from build123d import *

# Parameters (mm, degrees)
F0_R      = 57.15
F0_R_2    = 54.61
F1_DEPTH  = 12.7
F2_R      = 57.15
F2_R_2    = 55.88
F3_DEPTH  = 6.35
F5_DEPTH  = 25.4
F6_R      = 10.16
F8_R      = 57.3643246116
F8_R_2    = 56.3769302999
F9_DEPTH  = 5.08
F11_SIZE  = 3.81
F12_R     = 30.0710840357
F13_DEPTH = 5.08


# Not quite as in the source:
# - a fillet or chamfer that OpenCascade refuses, or shapes differently, is made with other operations: its cross-section is extruded or revolved along the edge and cut away or added
# - a feature names something its author has since deleted; it is built from what else it names


with BuildPart() as f1:
    # F0 (on Front) → F1 (new body)
    with BuildSketch(Plane.XZ):
        Circle(F0_R)
        Circle(F0_R_2, mode=Mode.SUBTRACT)
        Circle(F0_R_2)
    extrude(amount=F1_DEPTH)

    # F2 (on face) → F3 (join)
    with BuildSketch(Plane.XZ.offset(12.7)):
        Circle(F2_R)
        Circle(F2_R_2, mode=Mode.SUBTRACT)
    extrude(amount=F3_DEPTH)

    # F4 (on face) → F5 (join)
    with BuildSketch(Plane.XZ.offset(12.7)):
        with BuildLine():
            Line((9.1685925479, 8.7878843126), (12.836029567, 12.3030380376))
            ThreePointArc((12.836029567, 12.3030380376), (6.9778357566, 16.3535380928), (0, 17.78))
            Line((0, 17.78), (0, 12.7))
            ThreePointArc((0, 12.7), (4.9841683976, 11.6810986377), (9.1685925479, 8.7878843126))
        make_face()
        with BuildLine():
            ThreePointArc((12.3030380376, -12.836029567), (16.3535380928, -6.9778357566), (17.78, 0))
            Line((17.78, 0), (12.7, 0))
            ThreePointArc((12.7, 0), (11.6810986377, -4.9841683976), (8.7878843126, -9.1685925479))
            Line((8.7878843126, -9.1685925479), (12.3030380376, -12.836029567))
        make_face()
        with BuildLine():
            ThreePointArc((-12.836029567, -12.3030380376), (-6.9778357566, -16.3535380928), (0, -17.78))
            Line((0, -17.78), (0, -12.7))
            ThreePointArc((0, -12.7), (-4.9841683976, -11.6810986377), (-9.1685925479, -8.7878843126))
            Line((-9.1685925479, -8.7878843126), (-12.836029567, -12.3030380376))
        make_face()
        with BuildLine():
            Line((-8.7878843126, 9.1685925479), (-12.3030380376, 12.836029567))
            ThreePointArc((-12.3030380376, 12.836029567), (-16.3535380928, 6.9778357566), (-17.78, 0))
            Line((-17.78, 0), (-12.7, 0))
            ThreePointArc((-12.7, 0), (-11.6810986377, 4.9841683976), (-8.7878843126, 9.1685925479))
        make_face()
    extrude(amount=F5_DEPTH)

    # F6
    f6_edges = [f1.edges().sort_by_distance(p)[0] for p in [
        (-57.15, 0, 0),
    ]]
    fillet(f6_edges, radius=F6_R)

    # F8 (on offset) → F9 (cut)
    with BuildSketch(Plane.XZ.offset(12.7)):
        Circle(F8_R)
        Circle(F8_R_2, mode=Mode.SUBTRACT)
    extrude(amount=F9_DEPTH, mode=Mode.SUBTRACT)

    # F10: fillet of radius 3.81 on 3 edges, made by hand

    # F10_s1 → F10_t2 (revolve)
    with BuildSketch(Plane.XY):
        with BuildLine():
            ThreePointArc((56.3769302999, -15.0006856268), (56.5753652345, -13.7871380263), (57.15, -12.7))
            Line((57.15, -12.7), (57.089261394, -12.6539862875))
            ThreePointArc((57.089261394, -12.6539862875), (56.7634651499, -12.6238), (56.3769302999, -12.6238))
            Line((56.3769302999, -12.6238), (56.3007302999, -12.7))
            Line((56.3007302999, -12.7), (56.3007302999, -15.0006856268))
            Line((56.3007302999, -15.0006856268), (56.3769302999, -15.0006856268))
        make_face()
    revolve(axis=Axis((0, -12.7, 0), (0, -1, 0)))

    # F10_s3 → F10_t4 (revolve)
    with BuildSketch(Plane.XY):
        with BuildLine():
            ThreePointArc((57.15, -17.78), (56.5753652345, -16.6928619737), (56.3769302999, -15.4793143732))
            Line((56.3769302999, -15.4793143732), (56.3007302999, -15.4793143732))
            Line((56.3007302999, -15.4793143732), (56.3007302999, -17.78))
            Line((56.3007302999, -17.78), (56.3769302999, -17.8562))
            ThreePointArc((56.3769302999, -17.8562), (56.7634651499, -17.8562), (57.089261394, -17.8260137125))
            Line((57.089261394, -17.8260137125), (57.15, -17.78))
        make_face()
    revolve(axis=Axis((0, -17.78, 0), (0, -1, 0)))

    # F11
    f11_edges = [f1.edges().sort_by_distance(p)[0] for p in [
        (-16.353538, -38.1, 6.977836),
        (-6.977836, -38.1, -16.353538),
        (16.353538, -38.1, -6.977836),
        (6.977836, -38.1, 16.353538),
    ]]
    chamfer(f11_edges, length=F11_SIZE)

    # F12 (on face) → F13 (cut)
    with BuildSketch(Plane(origin=(0, 0, 0), x_dir=(-1, 0, 0), z_dir=(0, 1, 0))):
        Circle(F12_R)
    extrude(amount=-F13_DEPTH, mode=Mode.SUBTRACT)

    # F14: fillet of radius 86.36 on 1 edges, made by hand

    # F14_s1 → F14_t2 (revolve)
    with BuildSketch(Plane.XY):
        with BuildLine():
            ThreePointArc((-30.0710840357, 0), (-15.6993236042, -3.8005218602), (-0.8887057913, -5.08))
            Line((-0.8887057913, -5.08), (-30.0710840357, -5.08))
            Line((-30.0710840357, -5.08), (-30.0710840357, 0))
        make_face()
    revolve(axis=Axis((0, -5.08, 0), (0, 1, 0)))


solid = f1.part
CAD build for the part. Positions are in the model's coordinates, mm. A direction names the side the tool comes from. Give positions to 0.01 mm unless a question says otherwise; leave off trailing zeros. Order: outer loops, then holes, each group sorted by start corner. A loop starts at its lowest first (then second) coordinate and runs counter-clockwise, first axis right, second up. Notation, with made-up numbers: (-6.75, -23) -> (24.25, -23) arc R34 ccw to (24.25, 16) -> close; hole circle Ø10 at (60.25, 55.5). An arc over 180 degrees is marked (long way). Return JSON: item names as keys, results as strings.
Q1. Which spindle directions (+Z, -Z, +X, -X, +Y, -Y) get a long thin tool onto all of the face, cutting with end or side? Do faces 1 (the face through (-15, -25, 0)), 2 (the face through (5, -38.1, 12)). Say none if no direction does.
Working result:
{"face 1": "-Y", "face 2": "+Z, -Z, +X, -X, -Y"}
Q2. Flat gauge pins, fed straight in: pin 1 (12 mm diameter, centred on x = -30.5, y = -14, fed in from +Z); pin 2 (5.5 mm diameter, centred on y = -27, z = -14, fed in from +X); pin 3 (3 mm diameter, centred on x = 10.5, z = -41.5, fed in from -Y). Where does each tip first touch, or does it go through?
Working result:
{"pin 1": "z = 51.56", "pin 2": "x = 13.77", "pin 3": "y = -12.7"}
Q3. Drill centre lines: line 1 (Z direction, x = -6.5, y = -15.5); line 2 (Y direction, x = 39.5, z = -5.5); line 3 (X direction, y = -21, z = -11.5). Where is each one in solid material? Low to high.
Working result:
{"line 1": "-56 to -55.5, -16.55 to -10.91, 55.5 to 56", "line 2": "-12.7 to 0", "line 3": "-12 to -5.39, 11.02 to 13.56"}
Q4. Mould opens along Z. For faces 3 (the face through (12, -19.05, -55)), 4 (the face through (7.1, -23.3, 16.3)), 5 (the face through (14.541, -36.222, -6.302)) say: pulls with the +Z half, pulls with the -Z half, needs draft (parallel to the pull), parting line crosses it, or undercut.
Working result:
{"face 3": "needs draft", "face 4": "undercut", "face 5": "pulls with the -Z half"}
Q5. Saw through at A-A (y = -23.5). Write the cut outline in (x, z), then the cut area to 3 significant figures.
Working result:
{"outline": "(-17.78, 0) -> (-12.7, 0) arc R12.7 cw to (-8.79, 9.17) -> (-12.3, 12.84) arc R17.78 ccw to start; (-12.84, -12.3) arc R17.78 ccw to (0, -17.78) -> (0, -12.7) arc R12.7 cw to (-9.17, -8.79) -> close; (0, 12.7) arc R12.7 cw to (9.17, 8.79) -> (12.84, 12.3) arc R17.78 ccw to (0, 17.78) -> close; (8.79, -9.17) -> (12.3, -12.84) arc R17.78 ccw to (17.78, 0) -> (12.7, 0) arc R12.7 cw to start", "area": "250 mm²"}
